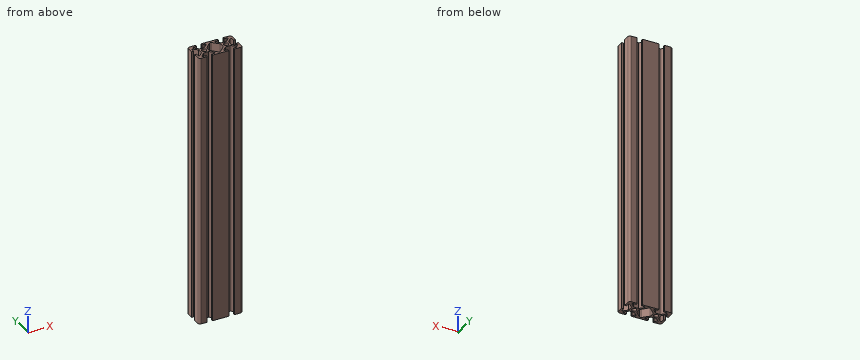
```python
from build123d import *

# Parameters (mm, degrees)
BOSS_EXTRUDE1_DEPTH = 125
BOSS_EXTRUDE2_DEPTH = 125
FILLET1_R           = 0.75
FILLET2_R           = 1.25


with BuildPart() as part:
    # Sketch3 → Boss-Extrude1 (new body, symmetric)
    with BuildSketch(Plane.XY):
        with BuildLine():
            Line((12.5, -10), (17.9, -10))
            ThreePointArc((17.9, -10), (19.38492424, -9.38492424), (20, -7.9))
            Line((20, -7.9), (20, -2.5))
            Line((20, -2.5), (18.213351365, -2.5))
            Line((18.213351365, -2.5), (18.213351365, -6.95))
            Line((18.213351365, -6.95), (13.6, -2.336648635))
            Line((13.6, -2.336648635), (13.6, 0))
            Line((13.6, 0), (12.15, 0))
            ThreePointArc((12.15, 0), (11.52027958, -1.52027958), (10, -2.15))
            Line((10, -2.15), (10, -3.6))
            Line((10, -3.6), (12.336648635, -3.6))
            Line((12.336648635, -3.6), (16.95, -8.213351365))
            Line((16.95, -8.213351365), (12.5, -8.213351365))
            Line((12.5, -8.213351365), (12.5, -10))
        make_face()
    extrude(amount=BOSS_EXTRUDE1_DEPTH, both=True)

    # Sketch4 → Boss-Extrude2 (add, symmetric)
    with BuildSketch(Plane.XY):
        with BuildLine():
            Line((10, -3.6), (7.663351365, -3.6))
            Line((7.663351365, -3.6), (3.05, -8.213351365))
            Line((3.05, -8.213351365), (7.5, -8.213351365))
            Line((7.5, -8.213351365), (7.5, -10))
            Line((7.5, -10), (0, -10))
            Line((0, -10), (0, -8.736648635))
            Line((0, -8.736648635), (6.4, -2.336648635))
            Line((6.4, -2.336648635), (6.4, 0))
            Line((6.4, 0), (7.85, 0))
            ThreePointArc((7.85, 0), (8.47972042, -1.52027958), (10, -2.15))
            Line((10, -2.15), (10, -3.6))
        make_face()
    extrude(amount=BOSS_EXTRUDE2_DEPTH, both=True)

    # Mirror1: part across plane


with BuildPart() as part_1:
    add(part.part)
    add(part.part.mirror(Plane(origin=(0, 0, 0), x_dir=(0, 0, 1), z_dir=(1, 0, 0))))

    # Mirror2: part across plane


with BuildPart() as part_2:
    add(part_1.part)
    add(part_1.part.mirror(Plane.ZX))

    # Fillet1
    fillet1_edges = [part_2.edges().sort_by_distance(p)[0] for p in [
        (18.213351365, 6.95, 0),
        (13.6, 2.336648635, 0),
        (12.336648635, 3.6, 0),
        (16.95, 8.213351365, 0),
        (3.05, 8.213351365, 0),
        (7.663351365, 3.6, 0),
        (-18.213351365, 6.95, 0),
        (-13.6, 2.336648635, 0),
        (-7.663351365, 3.6, 0),
        (-12.336648635, 3.6, 0),
        (-16.95, 8.213351365, 0),
        (-3.05, 8.213351365, 0),
        (16.95, -8.213351365, 0),
        (12.336648635, -3.6, 0),
        (13.6, -2.336648635, 0),
        (18.213351365, -6.95, 0),
        (3.05, -8.213351365, 0),
        (7.663351365, -3.6, 0),
        (-18.213351365, -6.95, 0),
        (-13.6, -2.336648635, 0),
        (-12.336648635, -3.6, 0),
        (-16.95, -8.213351365, 0),
        (-3.05, -8.213351365, 0),
        (-7.663351365, -3.6, 0),
    ]]
    fillet(fillet1_edges, radius=FILLET1_R)

    # Fillet2
    fillet2_edges = [part_2.edges().sort_by_distance(p)[0] for p in [
        (6.4, 2.336648635, 0),
        (0, 8.736648635, 0),
        (-6.4, 2.336648635, 0),
        (6.4, -2.336648635, 0),
        (-6.4, -2.336648635, 0),
        (0, -8.736648635, 0),
    ]]
    fillet(fillet2_edges, radius=FILLET2_R)


solid = part_2.part
```
The model under review builds one solid part; all positions refer to its coordinate system, in mm. Round coordinates to 2 decimals unless told otherwise and drop trailing zeros.
(1) We need section A-A on z = 44.5. Give the number of separate pieces and of enclosed holes in the cut face, and give its area (3 significant figures).
(2) Wall thickness on L1, parallel to Y at x = 10, z = 19; L2, parallel to Y at x = 7, z = 114; L3, parallel to Y at x = 6.5, z = 56: over which ranges is each line inside the solid? List them lowest first.
(3) Insertion check: pin 1 (2 mm diameter, centred on x = -19.5, z = -8, fed in from -Y); pin 2 (1.4 mm diameter, centred on y = -9, z = 26.5, fed in from +X); pin 3 (2 mm diameter, centred on y = 0.5, z = 49, fed in from +X); pin 4 (12 mm diameter, centred on x = 4, y = -1, fed in from +Z). Each pin has a flat end and moves straight along its axis. Give the tip position at first contact, or say it passes through.
Findings below:
1. separate pieces: 1
1. enclosed holes: 3
1. area: 324 mm2
2. L1: y = -3.6 to -2.15, 2.15 to 3.6
2. L2: y = -10 to -8.21, -4.26 to 4.26, 8.21 to 10
2. L3: y = -10 to -8.21, -4.76 to 4.76, 8.21 to 10
3. pin 1: stops at y = -9.91
3. pin 2: stops at x = 19.96
3. pin 3: stops at x = 13.6
3. pin 4: stops at z = 125
